Geometry check sheet. Reference: the model listing, model coordinates, mm. Face numbers are marked on the shaded views. Give positions to 0.01 mm unless a question says otherwise; leave off trailing zeros. Write each loop counter-clockwise with the first axis right and the second up, starting at its lowest first coordinate (ties: lowest second). Pieces come first, ordered by that corner, then holes.
(1) Depth check by flat-ended pin: P1, Ø12, axis at x = 813, y = 89, coming from the +Z side; P2, Ø12, axis at x = 373, y = 107, coming from the -Z side. Enter the tip coordinate at first touch or a pass-through.
(2) Cross-section at C-C (x = 1006.5). Record the boundary of the cut face in (y, z).
(3) Cross-section at B-B (y = 100). Record the boundary of the cut face in (x, z) (3 decimals).
(4) Cross-section at A-A (z = -91). Record the boundary of the cut face in (x, y) (3 decimals).
(5) Mould release check, pull along X, two halves, no side actions. Record for the marked faces 1, 2, 3 and 4: +X half, -X half, draft (parallel to the pull), parting line (faces both ways), or undercut.
(6) Thickness scan on line 1 along Z through (x, y) = (2, 25); line 2 along X through (y, z) = (100, -121.5) (3 decimals); line 3 along Y through (x, z) = (1.5, -127). Record the ranges inside material, lowest first.
```python
from build123d import *

# Parameters (mm, degrees)
SKETCH1_W           = 152.4
SKETCH1_H           = 152.4
BOSS_EXTRUDE1_DEPTH = 3.175
SKETCH2_W           = 4.7625
SKETCH2_H           = 152.4
BOSS_EXTRUDE2_DEPTH = 1206.5
SKETCH3_W           = 152.4
SKETCH3_H           = 152.4
BOSS_EXTRUDE3_DEPTH = 6.35
SKETCH4_R           = 5.55625
CUT_EXTRUDE1_DEPTH  = 1219.2


with BuildPart() as part:
    # Sketch1 → Boss-Extrude1 (new body)
    with BuildSketch(Plane(origin=(0, 0, 0), x_dir=(0, 0, -1), z_dir=(1, 0, 0))):
        with Locations((76.2, 76.2)):
            Rectangle(SKETCH1_W, SKETCH1_H)
    extrude(amount=BOSS_EXTRUDE1_DEPTH)

    # Sketch2 → Boss-Extrude2 (add)
    with BuildSketch(Plane(origin=(3.175, 0, 0), x_dir=(0, 0, -1), z_dir=(1, 0, 0))):
        with Locations((76.2, 76.2)):
            Rectangle(SKETCH2_W, SKETCH2_H)
    extrude(amount=BOSS_EXTRUDE2_DEPTH)

    # Sketch3 → Boss-Extrude3 (add)
    with BuildSketch(Plane(origin=(1209.675, 0, 0), x_dir=(0, 0, -1), z_dir=(1, 0, 0))):
        with Locations((76.2, 76.2)):
            Rectangle(SKETCH3_W, SKETCH3_H)
    extrude(amount=BOSS_EXTRUDE3_DEPTH)

    # Sketch4 → Cut-Extrude1 (cut)
    with BuildSketch(Plane.ZY):
        with Locations((-127, 127)):
            Circle(SKETCH4_R)
        with Locations((-25.4, 127)):
            Circle(SKETCH4_R)
        with Locations((-25.4, 25.4)):
            Circle(SKETCH4_R)
        with Locations((-127, 25.4)):
            Circle(SKETCH4_R)
    extrude(amount=-CUT_EXTRUDE1_DEPTH, mode=Mode.SUBTRACT)


solid = part.part
```
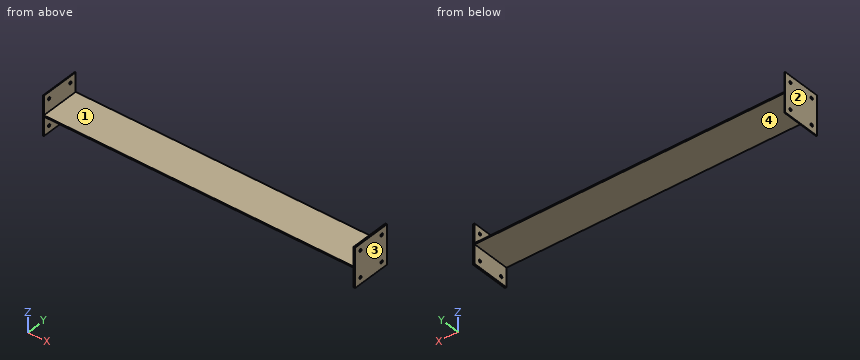
Reply:
1. P1: stops at z = -73.82
1. P2: stops at z = -78.58
2. outline: (0, -78.58) - (152.4, -78.58) - (152.4, -73.82) - (0, -73.82) - close
3. outline: (0, -152.4) - (3.175, -152.4) - (3.175, -78.581) - (1209.675, -78.581) - (1209.675, -152.4) - (1216.025, -152.4) - (1216.025, 0) - (1209.675, 0) - (1209.675, -73.819) - (3.175, -73.819) - (3.175, 0) - (0, 0) - close
4. outline: (0, 0) - (3.175, 0) - (3.175, 152.4) - (0, 152.4) - close; (1209.675, 0) - (1216.025, 0) - (1216.025, 152.4) - (1209.675, 152.4) - close
5. face 1: undercut
5. face 2: -X half
5. face 3: +X half
5. face 4: undercut
6. line 1: z = -152.4 to -132.54, -121.46 to -30.94, -19.86 to 0
6. line 2: x = 0 to 3.175, 1209.675 to 1216.025
6. line 3: y = 0 to 19.84, 30.96 to 121.44, 132.56 to 152.4
